Geometry: final body of the model. Coordinates: model frame, mm. Round coordinates to 2 decimals unless told otherwise and drop trailing zeros. Loops run counter-clockwise (first coordinate to the right, second up) from the corner with the lowest first, then second, coordinate; pieces in that order, holes last. Notation, with made-up numbers: (-25, 76) -> (32, 76) arc R23 ccw to (32, 111) -> close; hole circle Ø4 at (2.25, 77). An arc over 180 degrees is marked (long way). Answer in a Markdown table with one row per item.
```python
from build123d import *

# Parameters (mm, degrees)
SKETCH_R     = 8
SKETCH_R_2   = 3.2
SKETCH_R_3   = 4
SKETCH_R_4   = 1.8
PAD_DEPTH    = 1.6
SKETCH001_W  = 4.041902
SKETCH001_H  = 2.18935
POCKET_DEPTH = 5


with BuildPart() as part:
    # Sketch → Pad (new body)
    with BuildSketch(Plane.XY):
        with BuildLine():
            ThreePointArc((-15.710509, 39.802188), (-22, 46.091679), (-28.289491, 39.802188))
            Line((-28.289491, 39.802188), (-30, 39.802188))
            Line((-30, 39.802188), (-30, 64.895162))
            Line((-30, 64.895162), (30, 64.895162))
            Line((30, 33.895162), (30, 64.895162))
            Line((30, 33.895162), (18, 33.895162))
            Line((18, 33.895162), (18, 15.895162))
            Line((18, 15.895162), (30, 15.895162))
            Line((30, 15.895162), (30, -65.104838))
            Line((30, -65.104838), (-12, -65.104838))
            Line((-12, -49.414836), (-12, -65.104838))
            Line((-12, -8.197812), (-12, -49.414836))
            Line((-12, 39.802188), (-12, -8.197812))
            Line((-15.710509, 39.802188), (-12, 39.802188))
        make_face()
        with Locations((0, 39.802188)):
            Circle(SKETCH_R, mode=Mode.SUBTRACT)
        with Locations((22, 39.802188)):
            Circle(SKETCH_R_2, mode=Mode.SUBTRACT)
        with Locations((0, -60.104838)):
            Circle(SKETCH_R_3, mode=Mode.SUBTRACT)
        with Locations((25, -54.494838)):
            Circle(SKETCH_R_4, mode=Mode.SUBTRACT)
        with Locations((25, 59.895164)):
            Circle(SKETCH_R_4, mode=Mode.SUBTRACT)
        with Locations((-25, 59.895162)):
            Circle(SKETCH_R_4, mode=Mode.SUBTRACT)
    extrude(amount=PAD_DEPTH)

    # Sketch001 (on Face22 of Pad) → Pocket (cut)
    with BuildSketch(Plane.XY.offset(1.6)):
        with Locations((0, -64.491804)):
            Rectangle(SKETCH001_W, SKETCH001_H)
    extrude(amount=-POCKET_DEPTH, mode=Mode.SUBTRACT)


solid = part.part
```
Item 1: Draft query along Y for faces 1 (the face through (-21.86, 46.09, 0.79)), 2 (the face through (24.77, 61.68, 0.79)), 3 (the face through (7, 1, 0)). Return one class per face: pulls with the +Y half, pulls with the -Y half, needs draft (parallel to the pull), parting line crosses it, or undercut.
Answer:
| item | result |
|---|---|
| face 1 | pulls with the -Y half |
| face 2 | undercut |
| face 3 | needs draft |
Item 2: Line query: probe 1 along Y at (x, z) = (22, 0.7); probe 2 along Y at (x, z) = (0, 0.75); probe 3 along Y at (x, z) = (3.5, 0.9). Output: solid intervals per line, ascending. Write a range as [from, to].
Answer:
| item | result |
|---|---|
| probe 1 | y = [-65.1, 15.9], [33.9, 36.6], [43, 64.9] |
| probe 2 | y = [-56.1, 31.8], [47.8, 64.9] |
| probe 3 | y = [-65.1, -62.04], [-58.17, 32.61], [47, 64.9] |
Item 3: Cut plane D-D (x = -22). Output: boundary loops of the cut face in (y, z), then the cut area to 3 significant figures.
Answer:
| item | result |
|---|---|
| outline | (46.09, 0) -> (64.9, 0) -> (64.9, 1.6) -> (46.09, 1.6) -> close |
| area | 30.1 mm² |
Item 4: Cut plane A-A (x = 0). Output: boundary loops of the cut face in (y, z).
Answer:
| item | result |
|---|---|
| outline | (-56.1, 0) -> (31.8, 0) -> (31.8, 1.6) -> (-56.1, 1.6) -> close; (47.8, 0) -> (64.9, 0) -> (64.9, 1.6) -> (47.8, 1.6) -> close |
Item 5: Pin query (flat end, axial travel): pin 1 Ø0.5 at (y, z) = (23.5, 1) entering from +X; pin 2 Ø4 at (x, y) = (22, 39.8) entering from +Z. Return the tip coordinate at first contact, or that it passes through.
Answer:
| item | result |
|---|---|
| pin 1 | stops at x = 18 |
| pin 2 | passes through |
Item 6: Cut plane C-C (z = 0.7). Output: boundary loops of the cut face in (x, y).
Answer:
| item | result |
|---|---|
| outline | (-30, 39.8) -> (-28.29, 39.8) arc R6.29 cw to (-15.71, 39.8) -> (-12, 39.8) -> (-12, -65.1) -> (-2.02, -65.1) -> (-2.02, -63.56) arc R4 cw (long way) to (2.02, -63.56) -> (2.02, -65.1) -> (30, -65.1) -> (30, 15.9) -> (18, 15.9) -> (18, 33.9) -> (30, 33.9) -> (30, 64.9) -> (-30, 64.9) -> close; hole circle Ø3.6 at (-25, 59.9); hole circle Ø16 at (0, 39.8); hole circle Ø6.4 at (22, 39.8); hole circle Ø3.6 at (25, -54.49); hole circle Ø3.6 at (25, 59.9) |
Item 7: Cut plane B-B (x = 22). Output: boundary loops of the cut face in (y, z), then the cut area to 3 significant figures.
Answer:
| item | result |
|---|---|
| outline | (-65.1, 0) -> (15.9, 0) -> (15.9, 1.6) -> (-65.1, 1.6) -> close; (33.9, 0) -> (36.6, 0) -> (36.6, 1.6) -> (33.9, 1.6) -> close; (43, 0) -> (64.9, 0) -> (64.9, 1.6) -> (43, 1.6) -> close |
| area | 169 mm² |
